For this review, take the finished solid that the model builds, in its own axes (mm). A direction names the side the tool comes from. Coordinates: 2 decimals unless noted, no trailing zeros. Order: outer loops, then holes, each group sorted by start corner. A loop starts at its lowest first (then second) coordinate and runs counter-clockwise, first axis right, second up. Notation, with made-up numbers: M 27,81 L 44,81 A31 cw 44,106 Z; hole C 77.25,89 d7. An arc over 180 degrees is marked long. Use CSV: the item, a comma, the result in double quotes.
```python
from build123d import *

# Parameters (mm, degrees)
SKETCH1_W                 = 57.15
SKETCH1_H                 = 80.01
BOSS_EXTRUDE1_DEPTH       = 14.224
F_2_56_TAPPED_HOLE1_D     = 1.778
F_2_56_TAPPED_HOLE1_DEPTH = 5.588
F_2_56_TAPPED_HOLE1_TIP   = 0.53416509
CHAMFER1_SIZE             = 1.778
SKETCH4_W                 = 52.523792639
SKETCH4_H                 = 73.533309695
CUT_EXTRUDE1_DEPTH        = 2.54
SKETCH5_R                 = 3.175
BOSS_EXTRUDE2_DEPTH       = 5.842
CUT_EXTRUDE2_DEPTH        = 5.588
FILLET1_R                 = 2.794
CUT_EXTRUDE3_DEPTH        = 2.54


with BuildPart() as part:
    # Sketch1 → Boss-Extrude1 (new body)
    with BuildSketch(Plane(origin=(0, 0, 0), x_dir=(1, 0, 0), z_dir=(0, 1, 0))):
        Rectangle(SKETCH1_W, SKETCH1_H)
    extrude(amount=BOSS_EXTRUDE1_DEPTH)

    # #2-56 Tapped Hole1
    with Locations(Plane.XZ):
        with Locations((-20.6375, -37.9476), (-21.8694, 25.8318), (21.8694, 25.8318), (20.6375, -37.9476)):
            Hole(F_2_56_TAPPED_HOLE1_D / 2, depth=F_2_56_TAPPED_HOLE1_DEPTH)
            with Locations((0, 0, -(F_2_56_TAPPED_HOLE1_DEPTH + F_2_56_TAPPED_HOLE1_TIP / 2))):  # 118° drill point
                Cone(0, F_2_56_TAPPED_HOLE1_D / 2, F_2_56_TAPPED_HOLE1_TIP, mode=Mode.SUBTRACT)

    # Chamfer1
    chamfer1_edges = [part.edges().sort_by_distance(p)[0] for p in [
        (-28.575, 14.224, 0),
        (0, 14.224, 40.005),
        (28.575, 14.224, 0),
        (0, 14.224, -40.005),
    ]]
    chamfer(chamfer1_edges, length=CHAMFER1_SIZE)

    # Sketch4 → Cut-Extrude1 (cut)
    with BuildSketch(Plane.XZ):
        with Locations((-0.054148239, 0.758075358)):
            Rectangle(SKETCH4_W, SKETCH4_H)
    extrude(amount=-CUT_EXTRUDE1_DEPTH, mode=Mode.SUBTRACT)

    # Sketch5 → Boss-Extrude2 (add)
    with BuildSketch(Plane.XY.offset(40.005)):
        with Locations(Location((-12.7, 9.144, 0), (0, 0, 180))):
            Circle(SKETCH5_R)
        with Locations(Location((12.7, 9.144, 0), (0, 0, 180))):
            Circle(SKETCH5_R)
    extrude(amount=BOSS_EXTRUDE2_DEPTH)

    # Sketch6 → Cut-Extrude2 (cut)
    with BuildSketch(Plane(origin=(0, 14.224, 0), x_dir=(1, 0, 0), z_dir=(0, 1, 0))):
        with BuildLine():
            Line((18.796, 40.005), (18.796, 3.937))
            ThreePointArc((18.796, 3.937), (21.660202787, -2.977797213), (28.575, -5.842))
            Line((28.575, -5.842), (28.575, -0.508))
            ThreePointArc((28.575, -0.508), (25.431910358, 0.793910358), (24.13, 3.937))
            Line((24.13, 3.937), (24.13, 40.005))
            Line((24.13, 40.005), (18.796, 40.005))
        make_face()
        with BuildLine():
            Line((11.176, 40.005), (11.176, 3.937))
            ThreePointArc((11.176, 3.937), (16.272049114, -8.365950886), (28.575, -13.462))
            Line((28.575, -13.462), (28.575, -8.128))
            ThreePointArc((28.575, -8.128), (20.043756685, -4.594243315), (16.51, 3.937))
            Line((16.51, 3.937), (16.51, 40.005))
            Line((16.51, 40.005), (11.176, 40.005))
        make_face()
        with BuildLine():
            Line((28.575, -15.748), (28.575, -21.082))
            ThreePointArc((28.575, -21.082), (10.883895441, -13.754104559), (3.556, 3.937))
            ThreePointArc((3.556, 3.937), (2.514471714, 6.451471714), (0, 7.493))
            Line((0, 7.493), (0, 12.827))
            ThreePointArc((0, 12.827), (6.286179285, 10.223179285), (8.89, 3.937))
            ThreePointArc((8.89, 3.937), (14.655603012, -9.982396988), (28.575, -15.748))
        make_face()
    cut_extrude2 = extrude(amount=-CUT_EXTRUDE2_DEPTH, mode=Mode.SUBTRACT)

    # Mirror1: Cut-Extrude2 across plane
    add(cut_extrude2.mirror(Plane(origin=(0, 0, 0), x_dir=(0, 0, 1), z_dir=(1, 0, 0))), mode=Mode.SUBTRACT)

    # Fillet1
    # the kernel refuses this fillet: 2.794 mm, written as the material it adds along each edge
    with BuildSketch(Plane(origin=(-28.575, 8.636, -3.937), x_dir=(1, 0, 0), z_dir=(0, 0, -1))) as fillet1_piece_1:
        with BuildLine():
            CenterArc((9.779 - FILLET1_R, -FILLET1_R), FILLET1_R, 0, 90)
            Line((9.779, -FILLET1_R), (9.779, 0))
            Line((9.779, 0), (9.779 - FILLET1_R, 0))
        make_face()
    revolve(axis=Axis((-28.575, 8.636, -3.937), (0, -1, 0)), revolution_arc=90)
    with BuildSketch(Plane(origin=(-28.575, 8.636, -3.937), x_dir=(0, 0, 1), z_dir=(-1, 0, 0))) as fillet1_piece_2:
        with BuildLine():
            CenterArc((4.445 + FILLET1_R, FILLET1_R), FILLET1_R, 180, 90)
            Line((4.445 + FILLET1_R, 0), (4.445, 0))
            Line((4.445, 0), (4.445, FILLET1_R))
        make_face()
    revolve(axis=Axis((-28.575, 8.636, -3.937), (0, 1, 0)), revolution_arc=90)
    with BuildSketch(Plane(origin=(-28.575, 8.636, -3.937), x_dir=(0, 0, 1), z_dir=(-1, 0, 0))) as fillet1_piece_3:
        with BuildLine():
            CenterArc((12.065 + FILLET1_R, FILLET1_R), FILLET1_R, 180, 90)
            Line((12.065 + FILLET1_R, 0), (12.065, 0))
            Line((12.065, 0), (12.065, FILLET1_R))
        make_face()
    revolve(axis=Axis((-28.575, 8.636, -3.937), (0, 1, 0)), revolution_arc=90)
    with BuildSketch(Plane(origin=(-28.575, 8.636, -3.937), x_dir=(1, 0, 0), z_dir=(0, 0, -1))) as fillet1_piece_4:
        with BuildLine():
            CenterArc((17.399 - FILLET1_R, -FILLET1_R), FILLET1_R, 0, 90)
            Line((17.399, -FILLET1_R), (17.399, 0))
            Line((17.399, 0), (17.399 - FILLET1_R, 0))
        make_face()
    revolve(axis=Axis((-28.575, 8.636, -3.937), (0, -1, 0)), revolution_arc=90)
    with BuildSketch(Plane(origin=(28.575, 8.636, -3.937), x_dir=(0, 0, 1), z_dir=(1, 0, 0))) as fillet1_piece_5:
        with BuildLine():
            CenterArc((25.019 - FILLET1_R, -FILLET1_R), FILLET1_R, 0, 90)
            Line((25.019, -FILLET1_R), (25.019, 0))
            Line((25.019, 0), (25.019 - FILLET1_R, 0))
        make_face()
    revolve(axis=Axis((28.575, 8.636, -3.937), (0, -1, 0)), revolution_arc=90)
    with BuildSketch(Plane(origin=(0, 8.636, -3.937), x_dir=(-1, 0, 0), z_dir=(0, 0, 1))) as fillet1_piece_6:
        with BuildLine():
            CenterArc((3.556 + FILLET1_R, -FILLET1_R), FILLET1_R, 90, 90)
            Line((3.556, -FILLET1_R), (3.556, 0))
            Line((3.556, 0), (3.556 + FILLET1_R, 0))
        make_face()
    revolve(axis=Axis((0, 8.636, -3.937), (0, -1, 0)), revolution_arc=180)
    with BuildSketch(Plane(origin=(28.575, 8.636, -3.937), x_dir=(-1, 0, 0), z_dir=(0, 0, -1))) as fillet1_piece_7:
        with BuildLine():
            CenterArc((19.685 + FILLET1_R, FILLET1_R), FILLET1_R, 180, 90)
            Line((19.685 + FILLET1_R, 0), (19.685, 0))
            Line((19.685, 0), (19.685, FILLET1_R))
        make_face()
    revolve(axis=Axis((28.575, 8.636, -3.937), (0, 1, 0)), revolution_arc=90)
    with BuildSketch(Plane(origin=(-28.575, 8.636, -3.937), x_dir=(1, 0, 0), z_dir=(0, 0, -1))) as fillet1_piece_8:
        with BuildLine():
            CenterArc((19.685 + FILLET1_R, -FILLET1_R), FILLET1_R, 90, 90)
            Line((19.685 + FILLET1_R, 0), (19.685, 0))
            Line((19.685, 0), (19.685, -FILLET1_R))
        make_face()
    revolve(axis=Axis((-28.575, 8.636, -3.937), (0, -1, 0)), revolution_arc=90)
    with BuildSketch(Plane(origin=(28.575, 8.636, -3.937), x_dir=(0, 0, 1), z_dir=(1, 0, 0))) as fillet1_piece_9:
        with BuildLine():
            CenterArc((12.065 + FILLET1_R, -FILLET1_R), FILLET1_R, 90, 90)
            Line((12.065, -FILLET1_R), (12.065, 0))
            Line((12.065, 0), (12.065 + FILLET1_R, 0))
        make_face()
    revolve(axis=Axis((28.575, 8.636, -3.937), (0, -1, 0)), revolution_arc=90)
    with BuildSketch(Plane(origin=(28.575, 8.636, -3.937), x_dir=(-1, 0, 0), z_dir=(0, 0, -1))) as fillet1_piece_10:
        with BuildLine():
            CenterArc((17.399 - FILLET1_R, FILLET1_R), FILLET1_R, 270, 90)
            Line((17.399 - FILLET1_R, 0), (17.399, 0))
            Line((17.399, 0), (17.399, FILLET1_R))
        make_face()
    revolve(axis=Axis((28.575, 8.636, -3.937), (0, 1, 0)), revolution_arc=90)
    with BuildSketch(Plane(origin=(28.575, 8.636, -3.937), x_dir=(-1, 0, 0), z_dir=(0, 0, -1))) as fillet1_piece_11:
        with BuildLine():
            CenterArc((9.779 - FILLET1_R, FILLET1_R), FILLET1_R, 270, 90)
            Line((9.779 - FILLET1_R, 0), (9.779, 0))
            Line((9.779, 0), (9.779, FILLET1_R))
        make_face()
    revolve(axis=Axis((28.575, 8.636, -3.937), (0, 1, 0)), revolution_arc=90)
    with BuildSketch(Plane(origin=(28.575, 8.636, -3.937), x_dir=(0, 0, 1), z_dir=(1, 0, 0))) as fillet1_piece_12:
        with BuildLine():
            CenterArc((4.445 + FILLET1_R, -FILLET1_R), FILLET1_R, 90, 90)
            Line((4.445, -FILLET1_R), (4.445, 0))
            Line((4.445, 0), (4.445 + FILLET1_R, 0))
        make_face()
    revolve(axis=Axis((28.575, 8.636, -3.937), (0, -1, 0)), revolution_arc=90)
    with BuildSketch(Plane(origin=(-18.796, 8.636, -40.005), x_dir=(-1, 0, 0), z_dir=(0, 0, 1)), Plane(origin=(-11.176, 8.636, -40.005), x_dir=(-1, 0, 0), z_dir=(0, 0, 1)), Plane(origin=(11.176, 8.636, -40.005), x_dir=(0, 1, 0), z_dir=(0, 0, 1)), Plane(origin=(18.796, 8.636, -40.005), x_dir=(0, 1, 0), z_dir=(0, 0, 1))) as fillet1_piece_13:
        with BuildLine():
            CenterArc((FILLET1_R, -FILLET1_R), FILLET1_R, 90, 90)
            Line((0, -FILLET1_R), (0, 0))
            Line((0, 0), (FILLET1_R, 0))
        make_face()
    extrude(amount=36.068)
    with BuildSketch(Plane(origin=(-24.13, 8.636, -3.937), x_dir=(0, 1, 0), z_dir=(0, 0, -1)), Plane(origin=(-16.51, 8.636, -3.937), x_dir=(0, 1, 0), z_dir=(0, 0, -1)), Plane(origin=(16.51, 8.636, -3.937), x_dir=(-1, 0, 0), z_dir=(0, 0, -1)), Plane(origin=(24.13, 8.636, -3.937), x_dir=(-1, 0, 0), z_dir=(0, 0, -1))) as fillet1_piece_14:
        with BuildLine():
            CenterArc((FILLET1_R, FILLET1_R), FILLET1_R, 180, 90)
            Line((0, FILLET1_R), (0, 0))
            Line((0, 0), (FILLET1_R, 0))
        make_face()
    extrude(amount=36.068)
    with BuildSketch(Plane(origin=(-28.575, 8.636, -3.937), x_dir=(0, 0, 1), z_dir=(-1, 0, 0))) as fillet1_piece_15:
        with BuildLine():
            CenterArc((25.019 - FILLET1_R, FILLET1_R), FILLET1_R, 270, 90)
            Line((25.019, FILLET1_R), (25.019, 0))
            Line((25.019, 0), (25.019 - FILLET1_R, 0))
        make_face()
    revolve(axis=Axis((-28.575, 8.636, -3.937), (0, 1, 0)), revolution_arc=90)
    with BuildSketch(Plane(origin=(0, 8.636, -3.937), x_dir=(1, 0, 0), z_dir=(0, 0, 1))) as fillet1_piece_16:
        with BuildLine():
            CenterArc((8.89 - FILLET1_R, FILLET1_R), FILLET1_R, 270, 90)
            Line((8.89 - FILLET1_R, 0), (8.89, 0))
            Line((8.89, 0), (8.89, FILLET1_R))
        make_face()
    revolve(axis=Axis((0, 8.636, -3.937), (0, 1, 0)), revolution_arc=180)

    # Sketch7 → Cut-Extrude3 (cut)
    with BuildSketch(Plane(origin=(0, 14.224, 0), x_dir=(1, 0, 0), z_dir=(0, 1, 0))):
        Polygon((-3.141927936, -24.288971493), (-3.141927936, -14.763971493), (-2.962570965, -14.763971493), (3.330187448, -22.260711276), (3.330187448, -14.763971493), (4.18499514, -14.763971493), (4.18499514, -24.288971493), (3.990373746, -24.288971493), (-2.287120244, -16.809404185), (-2.287120244, -24.288971493), align=None)
    extrude(amount=-CUT_EXTRUDE3_DEPTH, mode=Mode.SUBTRACT)


solid = part.part
```
Item 1: Add section A-A on y = 3.75. State the section outline as (x, z) points (1 decimal).
Solutions:
outline,"M -28.6,-40 L 28.6,-40 L 28.6,40 L -28.6,40 Z; hole C -21.9,25.8 d1.8; hole C -20.6,-37.9 d1.8; hole C 20.6,-37.9 d1.8; hole C 21.9,25.8 d1.8"
Item 2: For faces 5 (the face through (13.113, 5.996, 42.885)), 6 (the face through (18, 14.224, -14)), 7 (the face through (21.585, 12.847, 2.901)), 8 (the face through (15.757, 9.521, -21.719)), 9 (the face through (0, 6, -40.005)), list the 3-axis set-ups (+Z, -Z, +X, -X, +Y, -Y) from which the entire face can be reached by the end or side of a thin tool; tool diameter is ignored.
Solutions:
face 5,"+Z"
face 6,"+Z, -Z, +X, -X, +Y"
face 7,"+Y"
face 8,"-Z, +Y"
face 9,"-Z, +X, -X, +Y, -Y"
Item 3: To check wall thickness, follow line 1 along X through (y, z) = (1, 17) (3 decimals); line 2 along X through (y, z) = (10.25, -16.5) (3 decimals); line 3 along Z through (x, y) = (-10, 2) (3 decimals). State the ranges of each line that lie inside material, in increasing order. Write a range as [from, to].
Solutions:
line 1,"[-28.575, -26.316], [26.208, 28.575]"
line 2,"[-28.575, -23.869], [-19.057, -16.249], [-11.437, 11.437], [16.249, 19.057], [23.869, 28.575]"
line 3,"[-40.005, -36.009], [37.525, 40.005]"
Item 4: Draft analysis for pull direction X (two halves, no side actions). For faces 1 (the face through (27.7, 13.32, 30.64)), 2 (the face through (-10.36, 7, 42.89)), 3 (the face through (-27.67, 13.35, 30.64)), 4 (the face through (17.64, 13.35, -39.1)), state which applies: released by +X, released by -X, zero draft, split by the parting line, or undercut.
Solutions:
face 1,"released by +X"
face 2,"undercut"
face 3,"released by -X"
face 4,"zero draft"
Item 5: Clearance check with flat-ended pins moving along their axes: pin 1 Ø8 at (x, z) = (-22, -13) entering from +Y; pin 2 Ø0.8 at (y, z) = (13, -29) entering from -X; pin 3 Ø3 at (x, z) = (21.87, 25.83) entering from -Y; pin 4 Ø0.8 at (y, z) = (13, -17.5) entering from +X. State where each tip first meets the part, or that it passes through.
Solutions:
pin 1,"y = 14.22"
pin 2,"x = -28.42"
pin 3,"y = 2.54"
pin 4,"x = 28.42"
